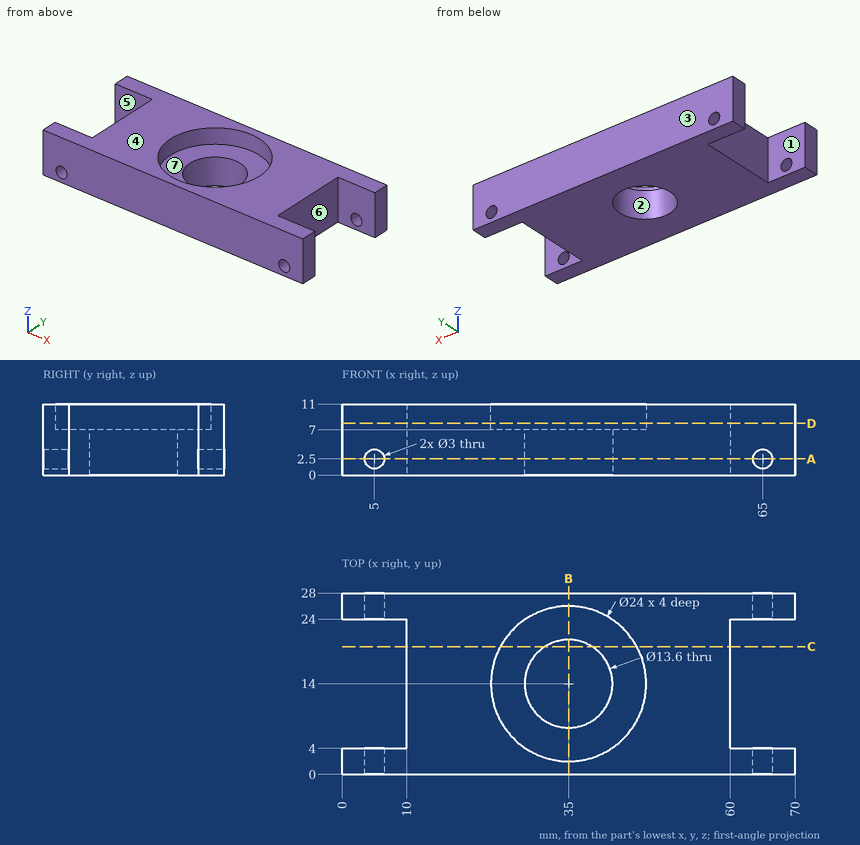
Answer from the drawing. Dimensions are ordinates in mm from the lowest x, y and z of the part. A direction names the side the tool comes from. Round coordinates to 2 decimals unless told otherwise and drop trailing zeros. Loops run counter-clockwise (first coordinate to the right, second up) from the corner with the lowest first, then second, coordinate; pieces in that order, holes last.
1) A cutting plane is placed at A-A on z = 2.5. Give the number of separate pieces and of enclosed holes in the cut face, plus the area to 3 significant figures.
Outcome:
separate pieces: 5
enclosed holes: 1
area: 1,370 mm2
2) A cutting plane is placed at C-C on y = 19.75. Determine the outline of the cut face in (x, z).
Outcome:
outline: (10, 0) - (31.37, 0) - (31.37, 7) - (24.47, 7) - (24.47, 11) - (10, 11) - close; (38.63, 0) - (60, 0) - (60, 11) - (45.53, 11) - (45.53, 7) - (38.63, 7) - close
3) For a pull along Y with two mould halves and no side action, classify the marked faces 1, 2, 3 and 4 as released by +Y, released by -Y, zero draft, split by the parting line, or undercut.
Outcome:
face 1: undercut
face 2: undercut
face 3: released by +Y
face 4: zero draft
4) Consider line 1 (X direction, y = 26.1, z = 2.5); line 2 (Y direction, x = 66, z = 4.25); line 3 (Z direction, x = 65, y = 24.9). Determine where each line is inside the solid, lowest interval first.
Outcome:
line 1: x = 0 to 3.5, 6.5 to 63.5, 66.5 to 70
line 2: y = 0 to 4, 24 to 28
line 3: z = 0 to 1, 4 to 11
5) A cutting plane is placed at D-D on z = 8. Determine the outline of the cut face in (x, y), plus the area to 3 significant figures.
Outcome:
outline: (0, 0) - (70, 0) - (70, 4) - (60, 4) - (60, 24) - (70, 24) - (70, 28) - (0, 28) - (0, 24) - (10, 24) - (10, 4) - (0, 4) - close; hole circle Ø24 at (35, 14)
area: 1,110 mm2
6) A cutting plane is placed at B-B on x = 35. Determine the outline of the cut face in (y, z), plus the area to 3 significant figures.
Outcome:
outline: (0, 0) - (7.2, 0) - (7.2, 7) - (2, 7) - (2, 11) - (0, 11) - close; (20.8, 0) - (28, 0) - (28, 11) - (26, 11) - (26, 7) - (20.8, 7) - close
area: 117 mm2
7) For the marked faces 5, 6 and 7, determine the directions among +Z, -Z, +X, -X, +Y, -Y from which every point of the face is accessible in a straight line to the end or side of a thin tool.
Outcome:
face 5: +Z, -Z, -X
face 6: +Z, -Z, +X
face 7: +Z
8) Given P1, Ø8, axis at x = 35, y = 14, coming from the +Z side; P2, Ø1.5, axis at x = 45.5, y = 19.5, coming from the +Z side; P3, Ø3.5, axis at y = 16.5, z = 7.5, coming from the +X side, each flat-ended and moving along its own axis, determine where each tip first touches the part or whether it passes through.
Outcome:
P1: passes through
P2: stops at z = 11
P3: stops at x = 60
